from build123d import *

# Parameters (mm, degrees)
SALIENTE_EXTRUIR1_DEPTH = 25.4
CROQUIS4_R              = 1.5
CROQUIS4_W              = 5.75
CROQUIS4_H              = 6.7
CORTAR_EXTRUIR3_DEPTH   = 29.45013181


with BuildPart() as part:
    # Croquis1 → Saliente-Extruir1 (new body)
    with BuildSketch(Plane.XY):
        with BuildLine():
            Line((0, -2.25), (12, -2.25))
            Line((12, -2.25), (12, -1.25))
            Line((12, -1.25), (1.870828693, -1.25))
            Line((1.870828693, -1.25), (0, -1.25))
            ThreePointArc((0, -1.25), (-0.883883476, 0.883883476), (1.25, 0))
            Line((1.25, 0), (1.25, -0.25))
            Line((1.25, -0.25), (2.236067977, -0.25))
            Line((2.236067977, -0.25), (2.25, -0.25))
            Line((2.25, -0.25), (2.25, 0))
            ThreePointArc((2.25, 0), (-1.590990258, 1.590990258), (0, -2.25))
        make_face()
    extrude(amount=SALIENTE_EXTRUIR1_DEPTH)

    # Croquis4 → Cortar-Extruir3 (cut, through all)
    with BuildSketch(Plane.XZ.offset(2.25)):
        with Locations(Location((8.5, 20.2, 0), (0, 0, 270))):
            Circle(CROQUIS4_R)
        with Locations(Location((8.5, 5.2, 0), (0, 0, 270))):
            Circle(CROQUIS4_R)
        with Locations((0.625, 22.05)):
            Rectangle(CROQUIS4_W, CROQUIS4_H)
        with Locations((0.625, 3.35)):
            Rectangle(CROQUIS4_W, CROQUIS4_H)
    extrude(amount=-CORTAR_EXTRUIR3_DEPTH, mode=Mode.SUBTRACT)


solid = part.part
Build history of the part. All positions in model axes, mm. A direction names the side the tool comes from. Give positions to 0.01 mm unless a question says otherwise; leave off trailing zeros. Loops run counter-clockwise (first coordinate to the right, second up) from the corner with the lowest first, then second, coordinate; pieces in that order, holes last. Notation, with made-up numbers: (21, 50.5) - (67, 50.5) arc R24 cw to (67, 86.5) - close; hole circle Ø5 at (57.5, -28.75). An arc over 180 degrees is marked (long way). Write item = value, one per line. Start each with the question number.
1) Band-saw the part on A-A on x = 8.5. Give the cut face in (y, z), plus the area to 3 significant figures.
2) Pull direction X, two halves, no side cores. Call faces 5 (the flat face through (6, -2.25, 13)), 6 (the flat face through (12, -2, 13)), 7 (the cylindrical face through (7.036, -1.757, 20.525)): +X half, -X half, draft (parallel to the pull), parting line (faces both ways), or undercut.
3) Band-saw the part on B-B on z = 5.2. Give the cut face in (x, y), plus the area to 3 significant figures.
4) Band-saw the part on D-D on z = 8.5. Give the cut face in (x, y), plus the area to 3 significant figures.
5) Probe probe 1 along Y at (x, z) = (0, 15); probe 2 along X at (y, z) = (-1.9, 5.2); probe 3 along Z at (x, y) = (8, -1.3). List the from-to ranges inside material, lowest first. Write a range as from..to.
6) Drop flat-ended pins along their axis: pin 1 Ø1.1 at (y, z) = (-1.5, 3.5) entering from -X; pin 2 Ø6 at (x, z) = (6, 7) entering from +Y; pin 3 Ø1.5 at (x, y) = (0, 0) entering from +Z; pin 4 Ø1.5 at (x, z) = (2, 15.5) entering from +Y. Give the stop position or say it passes through.
7) Band-saw the part on C-C on y = 0.35. Give the cut face in (x, z).
8) Tool access for faces 1 (the flat face through (6, -1.25, 13)), 2 (the flat face through (3.5, -2, 22)), 3 (the flat face through (8, -2, 25.4)), 4 (the flat face through (3.5, -2, 3)): list every direction of +Z, -Z, +X, -X, +Y, -Y with a clear straight run to the whole face (end or side of a thin tool).
Final values:
q1.outline = (-2.25, 0) - (-1.25, 0) - (-1.25, 3.7) - (-2.25, 3.7) - close; (-2.25, 6.7) - (-1.25, 6.7) - (-1.25, 18.7) - (-2.25, 18.7) - close; (-2.25, 21.7) - (-1.25, 21.7) - (-1.25, 25.4) - (-2.25, 25.4) - close
q1.area = 19.4 mm²
q2.face_5 = draft
q2.face_6 = +X half
q2.face_7 = undercut
q3.outline = (3.5, -2.25) - (7, -2.25) - (7, -1.25) - (3.5, -1.25) - close; (10, -2.25) - (12, -2.25) - (12, -1.25) - (10, -1.25) - close
q3.area = 5.50 mm²
q4.outline = (0, -2.25) - (12, -2.25) - (12, -1.25) - (0, -1.25) arc R1.25 cw (long way) to (1.25, 0) - (1.25, -0.25) - (2.25, -0.25) - (2.25, 0) arc R2.25 ccw (long way) to start
q4.area = 20.5 mm²
q5.probe_1 = -2.25..-1.25, 1.25..2.25
q5.probe_2 = 3.5..7, 10..12
q5.probe_3 = 0..3.79, 6.61..18.79, 21.61..25.4
q6.pin_1 = 3.5
q6.pin_2 = -1.25
q6.pin_3 = through
q6.pin_4 = 1.87
q7.outline = (-2.22, 6.7) - (-1.2, 6.7) - (-1.2, 18.7) - (-2.22, 18.7) - close; (1.2, 6.7) - (2.22, 6.7) - (2.22, 18.7) - (1.2, 18.7) - close
q8.face_1 = +Z, -Z, +X
q8.face_2 = +Z, -X, +Y, -Y
q8.face_3 = +Z, +X, -X, +Y, -Y
q8.face_4 = -Z, -X, +Y, -Y
